Design review of the part built by this model. Coordinates are the model's own, in mm. A direction names the side the tool comes from. Coordinates: 2 decimals unless noted, no trailing zeros. Order: outer loops, then holes, each group sorted by start corner. A loop starts at its lowest first (then second) coordinate and runs counter-clockwise, first axis right, second up. Notation, with made-up numbers: (-25.75, -19) - (-17.75, -19) arc R16 ccw to (-17.75, 3) - close; hole circle Ø7 at (-23, -4.5). An arc over 180 degrees is marked (long way). Write item = value, one per line. Start each with the question number.
```python
from build123d import *

# Parameters (mm, degrees)
SKETCH1_R           = 1.5
BOSS_EXTRUDE1_DEPTH = 3
FILLET1_R           = 3
SCALE1_SCALE        = 0.888888889


with BuildPart() as part:
    # Sketch1 → Boss-Extrude1 (new body)
    with BuildSketch(Plane(origin=(0, 0, 0), x_dir=(1, 0, 0), z_dir=(0, 1, 0))):
        with BuildLine():
            ThreePointArc((3.16227766, 1.5), (-3.5, 0), (3.16227766, -1.5))
            Line((3.16227766, -1.5), (27.83772234, -1.5))
            ThreePointArc((27.83772234, -1.5), (34.5, 0), (27.83772234, 1.5))
            Line((27.83772234, 1.5), (3.16227766, 1.5))
        make_face()
        with Locations(Location((0, 0, 0), (0, 0, 270))):
            Circle(SKETCH1_R, mode=Mode.SUBTRACT)
        with Locations(Location((31, 0, 0), (0, 0, 270))):
            Circle(SKETCH1_R, mode=Mode.SUBTRACT)
    extrude(amount=BOSS_EXTRUDE1_DEPTH)

    # Fillet1
    fillet1_edges = [part.edges().sort_by_distance(p)[0] for p in [
        (27.83772234, 1.5, 1.5),
        (3.16227766, 1.5, 1.5),
        (3.16227766, 1.5, -1.5),
        (27.83772234, 1.5, -1.5),
    ]]
    fillet(fillet1_edges, radius=FILLET1_R)


with BuildPart() as part_1:
    # Scale1: scaled about (15.5, 1.5, 0)
    add(part.part.scale(SCALE1_SCALE).moved(Location((1.722222222, 0.166666667, 0))))


solid = part_1.part
```
Item 1: For line 1 (X direction, y = 2.3, z = 0); line 2 (Z direction, x = 10.5, y = 0.3); line 3 (X direction, y = 1.5, z = 2.75), list the stretches that pass through material, from the lowest coordinate up.
Item 2: For P1, Ø1.5, axis at x = 10, y = 2, coming from the -Z side; P2, Ø3.5, axis at x = 29.28, z = 0, coming from the +Y side, all flat-tipped, find the tip position at first contact; note any pin that passes through.
Item 3: Add section A-A on z = 0. Give the boundary of the cut face in (x, y).
Item 4: Mouldability with a two-part tool opening along X and no side actions: class faces 4 (the flat face through (15, 1, 1.333)), 5 (the flat face through (15, 0.167, 0)) as +X half, -X half, draft (parallel to the pull), parting line (faces both ways), or undercut.
Item 5: Add section B-B on y = 1.4. Give the boundary of the cut face in (x, z).
Item 6: Add section C-C on z = -2.5. Give the boundary of the cut face in (x, y).
Item 7: Add section D-D on x = 4.5. Give the boundary of the cut face in (y, z), plus the area to 3 significant figures.
Item 8: For faces 1 (the cylindrical face through (4.832, 1.519, 1.553)), 2 (the cylindrical face through (4.832, 1.519, -1.553)), 3 (the cylindrical face through (-1.387, 1.481, -0.104)), list the 3-axis set-ups (+Z, -Z, +X, -X, +Y, -Y) from which the entire face can be reached by the end or side of a thin tool; tool diameter is ignored.
Worked out:
q1.line_1 = -1.39 to 0.39, 3.06 to 27.94, 30.61 to 32.39
q1.line_2 = -1.33 to 1.33
q1.line_3 = 0.27 to 3.18, 27.82 to 30.73
q2.P1 = -1.33
q2.P2 = 2.83
q3.outline = (-1.39, 0.17) - (0.39, 0.17) - (0.39, 2.83) - (-1.39, 2.83) - close; (3.06, 0.17) - (27.94, 0.17) - (27.94, 2.83) - (3.06, 2.83) - close; (30.61, 0.17) - (32.39, 0.17) - (32.39, 2.83) - (30.61, 2.83) - close
q4.face_4 = undercut
q4.face_5 = draft
q5.outline = (3.97, -2.15) arc R2.67 cw to (5.89, -1.33) - (25.11, -1.33) arc R2.67 cw to (27.03, -2.15) arc R3.11 ccw (long way) to (27.03, 2.15) arc R2.67 cw to (25.11, 1.33) - (5.89, 1.33) arc R2.67 cw to (3.97, 2.15) arc R3.11 ccw (long way) to start; hole circle Ø2.67 at (1.72, 0); hole circle Ø2.67 at (29.28, 0)
q6.outline = (-0.13, 0.17) - (3.57, 0.17) - (3.57, 2.83) - (-0.13, 2.83) - close; (27.43, 0.17) - (31.13, 0.17) - (31.13, 2.83) - (27.43, 2.83) - close
q7.outline = (0.17, -1.73) - (2.83, -1.73) - (2.83, 1.73) - (0.17, 1.73) - close
q7.area = 9.20 mm2
q8.face_1 = +Z, +Y, -Y
q8.face_2 = -Z, +Y, -Y
q8.face_3 = +Y, -Y
